Build history of the part. All positions in model axes, mm. Face numbers are marked on the shaded views. A direction names the side the tool comes from. Coordinates: 2 decimals unless noted, no trailing zeros. Order: outer loops, then holes, each group sorted by start corner. A loop starts at its lowest first (then second) coordinate and runs counter-clockwise, first axis right, second up. Notation, with made-up numbers: (-15, 14.5) - (42, 14.5) arc R22 cw to (42, 39.5) - close; hole circle Ø10 at (-37, 34). An arc over 180 degrees is marked (long way). Return JSON: item names as keys, results as strings.
Autodesk Inventor part; units mm, degrees
ref_plane "YZ Plane" through (0, 0, 0) normal (1, 0, 0) x (0, 1, 0)
ref_plane "XZ Plane" through (0, 0, 0) normal (0, 1, 0) x (-1, 0, 0)
ref_plane "XY Plane" through (0, 0, 0) normal (0, 0, 1) x (1, 0, 0)
sketch "Sketch1" plane through (0, 0, 0) normal (0, 1, 0) x (-1, 0, 0)
  line L0 (-49.2125, 50.8) -> (49.2125, 50.8)
  line L1 (49.2125, 50.8) -> (49.2125, -50.8)
  line L2 (49.2125, -50.8) -> (-49.2125, -50.8)
  line L3 (-49.2125, -50.8) -> (-49.2125, 50.8)
  line L4 (-49.2125, 50.8) -> (49.2125, -50.8) construction
  line L5 (49.2125, 50.8) -> (-49.2125, -50.8) construction
  point P0 (0, 0)
  dimension "d0" = 98.425
  dimension "d1" = 101.6
extrude "Plate1" add sketch "Sketch1" along normal blind 0.7144
sketch "Sketch2" plane through (-49.2125, 0.7144, 50.0856) normal (0, 0, 1) x (1, 0, 0)
  line L0 (98.425, 0) -> (0, 0)
  line L1 (0, 0) -> (0, -98.425)
  line L2 (0, -98.425) -> (98.425, -98.425)
  line L3 (98.425, -98.425) -> (98.425, 0)
edge flange "Flange1" height 98.425 angle 90 thickness 0.7144 bend radius 0.7144 thickness toward (0, 0, 1) relief tear relief width 0.7144 relief depth 0.3572 edges at (0, 0, 50.8) wall of the first edge with corners at (49.2125, 0.7144, 50.0856) (-49.2125, 0.7144, 50.0856) (-49.2125, -97.7106, 50.0856) (49.2125, -97.7106, 50.0856)
bend "Bend1"
corner "Corner1"
sketch "Sketch3" plane through (0, 0.7144, 0) normal (0, 1, 0) x (1, 0, 0)
  line L0 (28.575, -28.575) -> (-28.575, -28.575)
  line L1 (-28.575, -28.575) -> (-28.575, 28.575)
  line L2 (-28.575, 28.575) -> (28.575, 28.575)
  line L3 (28.575, 28.575) -> (28.575, -28.575)
  line L4 (28.575, -28.575) -> (-28.575, 28.575) construction
  line L5 (-28.575, -28.575) -> (28.575, 28.575) construction
  point P0 (0, 0)
  dimension "d13" = 57.15
  dimension "d14" = 57.15
extrude "Extrusion1" cut sketch "Sketch3" against normal blind 0.7144
equation "\"d15\" = Thickness"
equation "\"d2\" = Thickness"
equation "\"d3\" = BendReliefWidth"
equation "\"d4\" = BendReliefDepth"
equation "\"d5\" = MinimumRemnant"
equation "\"d6\" = TransitionRadius"
equation "\"d9\" = BendRadius"
equation "\"d10\" = CornerReliefSize"
equation "\"d11\" = GapSize"
equation "\"d12\" = JacobiRadiusSize"
equation "\"BendRadius\" = Thickness"
equation "\"BendReliefWidth\" = Thickness"
equation "\"BendReliefDepth\" = 0.5 * Thickness"
equation "\"CornerReliefSize\" = 4 * Thickness"
equation "\"MinimumRemnant\" = 2 * Thickness"
equation "\"TransitionRadius\" = BendRadius"
equation "\"JacobiRadiusSize\" = BendRadius"
equation "\"GapSize\" = Thickness"
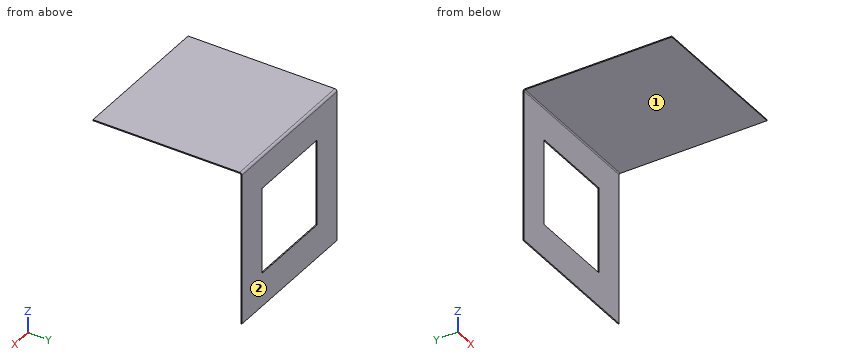
1. Probe L1, parallel to Y at x = 17.5, z = 40.5; L2, parallel to Z at x = 14.5, y = -77.5. List the from-to ranges inside material, lowest first.
Check values:
{"L1": "0 to 0.71", "L2": "50.09 to 50.8"}
2. Tool access for the marked faces 1 and 2: list every direction of +Z, -Z, +X, -X, +Y, -Y with a clear straight run to the whole face (end or side of a thin tool).
Check values:
{"face 1": "-Z, +X, -X, -Y", "face 2": "+Z, -Z, +X, -X, +Y"}
3. Cut at A-A on z = -13. Give the cut face in (x, y) (1 decimal).
Check values:
{"outline": "(-49.2, 0) - (-28.6, 0) - (-28.6, 0.7) - (-49.2, 0.7) - close; (28.6, 0) - (49.2, 0) - (49.2, 0.7) - (28.6, 0.7) - close"}
4. Cut at B-B on x = 7.5. Give the cut face in (y, z) (3 decimals), plus the area to 3 significant figures.
Check values:
{"outline": "(-97.711, 50.086) - (-0.714, 50.086) arc R0.714 cw to (0, 49.371) - (0, 28.575) - (0.714, 28.575) - (0.714, 49.371) arc R1.429 ccw to (-0.714, 50.8) - (-97.711, 50.8) - close; (0, -50.8) - (0.714, -50.8) - (0.714, -28.575) - (0, -28.575) - close", "area": "101 mm²"}
5. Drop flat-ended pins along their axis: pin 1 (6 mm diameter, centred on x = 26.5, y = -49, fed in from -Z); pin 2 (1 mm diameter, centred on x = 24, z = -35.5, fed in from -Y); pin 3 (12 mm diameter, centred on x = -19.5, z = 17, fed in from -Y). Give the stop position or say it passes through.
Check values:
{"pin 1": "z = 50.09", "pin 2": "y = 0", "pin 3": "through"}
6. Cut at D-D on z = 33.5. Give the cut face in (x, y).
Check values:
{"outline": "(-49.21, 0) - (49.21, 0) - (49.21, 0.71) - (-49.21, 0.71) - close"}
7. Cut at C-C on x = 43. Give the cut face in (y, z).
Check values:
{"outline": "(-97.71, 50.09) - (-0.71, 50.09) arc R0.71 cw to (0, 49.37) - (0, -50.8) - (0.71, -50.8) - (0.71, 49.37) arc R1.43 ccw to (-0.71, 50.8) - (-97.71, 50.8) - close"}
